from build123d import *

# Parameters (mm, degrees)
F0_W     = 17
F0_H     = 17
F1_DEPTH = 1.5
F2_W     = 2
F2_H     = 4
F3_DEPTH = 3
F4_R     = 1


with BuildPart() as f1:
    # F0 (on Top) → F1 (new body)
    with BuildSketch(Plane.XY):
        Rectangle(F0_W, F0_H)
    extrude(amount=F1_DEPTH)

    # F2 (on face) → F3 (join)
    with BuildSketch(Plane.XY.offset(1.5)):
        with BuildLine():
            ThreePointArc((-1, 2.5), (0, 1.5), (1, 2.5))
            Line((1, 2.5), (-1, 2.5))
        make_face()
        with Locations((0, 4.5)):
            Rectangle(F2_W, F2_H)
        with BuildLine():
            Line((-1, 6.5), (1, 6.5))
            ThreePointArc((1, 6.5), (0, 7.5), (-1, 6.5))
        make_face()
    extrude(amount=F3_DEPTH)

    # F4
    f4_edges = [f1.edges().sort_by_distance(p)[0] for p in [
        (-8.5, 8.5, 0.75),
        (-8.5, -8.5, 0.75),
        (8.5, 8.5, 0.75),
        (8.5, -8.5, 0.75),
    ]]
    fillet(f4_edges, radius=F4_R)


solid = f1.part
Build history of the part. All positions in model axes, mm. A direction names the side the tool comes from. Coordinates: 2 decimals unless noted, no trailing zeros. Write each loop counter-clockwise with the first axis right and the second up, starting at its lowest first coordinate (ties: lowest second). Pieces come first, ordered by that corner, then holes.
(1) Cut at D-D on y = -0.75. List the corners of the cut face in (x, z), and give its area (3 significant figures).
(2) Cut at C-C on z = 3.05. List the corners of the cut face in (x, y).
(3) Cut at A-A on y = 3.5. List the corners of the cut face in (x, z).
(4) Drill centre lines: line 1 (Z direction, x = 2, y = -0.5); line 2 (X direction, y = 6, z = 2.1). Where is each one in solid material? Low to high.
(5) Cut at B-B on x = 0. List the corners of the cut face in (y, z), and give its area (3 significant figures).
(6) 3-axis set-ups, long thin cutter, end or side, ignore diameter. For faces 1 (the cylindrical face through (0, 1.5, 3)), 2 (the cylindrical face through (0, 7.5, 3)), 3 (the flat face through (8.5, 0, 1)), 4 (the flat face through (1, 4, 3)), 5 (the flat face through (-1, 4, 3)): which of +Z, -Z, +X, -X, +Y, -Y reach the whole face in a straight line?
(7) Pin check, flat tips, straight feed: pin 1 Ø2 at (y, z) = (-2.5, 3) entering from -X; pin 2 Ø8.5 at (x, y) = (-3, 0) entering from +Z; pin 3 Ø0.9 at (y, z) = (5, 3) entering from -X. Stop position of each tip, or through.
Working result:
1. outline: (-8.5, 0) - (8.5, 0) - (8.5, 1.5) - (-8.5, 1.5) - close
1. area: 25.5 mm2
2. outline: (-1, 2.5) arc R1 ccw to (1, 2.5) - (1, 6.5) arc R1 ccw to (-1, 6.5) - close
3. outline: (-8.5, 0) - (8.5, 0) - (8.5, 1.5) - (1, 1.5) - (1, 4.5) - (-1, 4.5) - (-1, 1.5) - (-8.5, 1.5) - close
4. line 1: z = 0 to 1.5
4. line 2: x = -1 to 1
5. outline: (-8.5, 0) - (8.5, 0) - (8.5, 1.5) - (7.5, 1.5) - (7.5, 4.5) - (1.5, 4.5) - (1.5, 1.5) - (-8.5, 1.5) - close
5. area: 43.5 mm2
6. face 1: +Z, -Y
6. face 2: +Z, +Y
6. face 3: +Z, -Z, +X, +Y, -Y
6. face 4: +Z, +X, +Y, -Y
6. face 5: +Z, -X, +Y, -Y
7. pin 1: passes through
7. pin 2: stops at z = 4.5
7. pin 3: stops at x = -1
